from build123d import *

# Parameters (mm, degrees)
SKETCH1_W          = 75
SKETCH1_H          = 120
BASE_FLANGE1_DEPTH = 10
SKETCH7_R          = 2.5
CUT_EXTRUDE1_DEPTH = 10


# Sheet-metal steps are written as plain solids
with BuildPart() as part:
    # Sketch1 → Base-Flange1 (new body)
    with BuildSketch(Plane.XY):
        with Locations((37.5, 60)):
            Rectangle(SKETCH1_W, SKETCH1_H)
    extrude(amount=-BASE_FLANGE1_DEPTH)

    # Sketch7 → Cut-Extrude1 (cut)
    with BuildSketch(Plane.XY):
        with Locations((10, 110)):
            Circle(SKETCH7_R)
        with Locations((22.5, 7.5)):
            Circle(SKETCH7_R)
        with Locations(Location((52.5, 7.5, 0), (0, 0, 180))):
            Circle(SKETCH7_R)
        with Locations(Location((65, 110, 0), (0, 0, 180))):
            Circle(SKETCH7_R)
        Polygon((15, 105), (15, 41.062028891), (60, 105), align=None)
        Polygon((15, 15), (60, 15), (60, 78.937971109), align=None)
    extrude(amount=-CUT_EXTRUDE1_DEPTH, mode=Mode.SUBTRACT)


solid = part.part
Check sheet for the modelled part. Datum: model origin and axes. Units: mm. A direction names the side the tool comes from. Round coordinates to 2 decimals unless told otherwise and drop trailing zeros. Order: outer loops, then holes, each group sorted by start corner. A loop starts at its lowest first (then second) coordinate and runs counter-clockwise, first axis right, second up.
(1) Cross-section at D-D, the plane z = -5. Enter the section's corners in (x, y).
(2) Draft check along Y on faces 1 (the flat face through (37, 120, -5)), 2 (the flat face through (37, 61, -10)), 3 (the cylindrical face through (50.19, 8.46, -4.93)). Enter one of: pulls with the +Y half, pulls with the -Y half, needs draft (parallel to the pull), parting line crosses it, or undercut.
(3) Cross-section at B-B, the plane x = 65. Enter the section's corners in (y, z), and give its area (3 significant figures).
(4) Go/stop test with a flat-tipped pin: P1, Ø4, axis at x = 65, y = 110, coming from the -Z side. Record where the tip stops, or that it passes through.
(5) Cross-section at C-C, the plane y = 29. Enter the section's corners in (x, z).
(6) Cross-section at A-A, the plane y = 110. Enter the section's corners in (x, z).
(7) Access from +Z, -Z, +X, -X, +Y, -Y to the whole of each face (thin tool, end or side, straight path). Record for faces 4 (the flat face through (60, 47, -5)), 5 (the flat face through (75, 59, -5)).
(8) Scan lines: probe 1 along Y at (x, z) = (65, -4.5); probe 2 along Y at (x, z) = (22.5, -6.25); probe 3 along X at (y, z) = (52.5, -3.5). Record each from-to range of solid material in increasing order.
Check sheet entries:
1. outline: (0, 0) - (75, 0) - (75, 120) - (0, 120) - close; hole circle Ø5 at (10, 110); hole (15, 15) - (60, 15) - (60, 78.94) - close; hole (15, 41.06) - (60, 105) - (15, 105) - close; hole circle Ø5 at (22.5, 7.5); hole circle Ø5 at (52.5, 7.5); hole circle Ø5 at (65, 110)
2. face 1: pulls with the +Y half
2. face 2: needs draft
2. face 3: undercut
3. outline: (0, -10) - (107.5, -10) - (107.5, 0) - (0, 0) - close; (112.5, -10) - (120, -10) - (120, 0) - (112.5, 0) - close
3. area: 1,150 mm2
4. P1: passes through
5. outline: (0, -10) - (24.85, -10) - (24.85, 0) - (0, 0) - close; (60, -10) - (75, -10) - (75, 0) - (60, 0) - close
6. outline: (0, -10) - (7.5, -10) - (7.5, 0) - (0, 0) - close; (12.5, -10) - (62.5, -10) - (62.5, 0) - (12.5, 0) - close; (67.5, -10) - (75, -10) - (75, 0) - (67.5, 0) - close
7. face 4: +Z, -Z
7. face 5: +Z, -Z, +X, +Y, -Y
8. probe 1: y = 0 to 107.5, 112.5 to 120
8. probe 2: y = 0 to 5, 10 to 15, 25.66 to 51.72, 105 to 120
8. probe 3: x = 0 to 15, 23.05 to 41.39, 60 to 75
